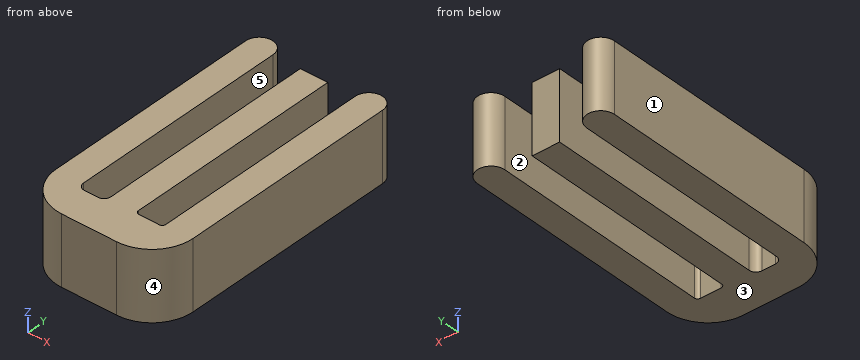
Autodesk Fusion 360 part; units mm, degrees
sketch "Sketch1" plane through (0, 0, 0) normal (0, 0, 1) x (1, 0, 0)
  line L0 (0, 0) -> (200, 0)
  line L1 (200, 0) -> (200, 200)
  line L2 (200, 200) -> (0, 200)
  line L3 (0, 200) -> (0, 0)
  line L4 (52.8009, 30) -> (52.8009, 190)
  line L5 (72.8009, 190) -> (72.8009, 30)
  line L6 (112.8009, 190) -> (112.8009, 30)
  line L7 (132.8009, 190) -> (132.8009, 30)
  line L8 (152.8009, 190) -> (152.8009, 30)
  line L9 (52.8009, 190) -> (152.8009, 190) construction
  arc A0 (72.8009, 190) -> (52.8009, 190) centre (62.8009, 190) ccw
  arc A1 (152.8009, 190) -> (132.8009, 190) centre (142.8009, 190) ccw
  line L10 (92.8009, 190) -> (92.8009, 30)
  arc A2 (72.8009, 30) -> (92.8009, 30) centre (82.8009, 30) ccw construction
  arc A3 (112.8009, 30) -> (132.8009, 30) centre (122.8009, 30) ccw construction
  arc A4 (112.8009, 190) -> (92.8009, 190) centre (102.8009, 190) ccw construction
  arc A5 (52.8009, 30) -> (82.8009, 0) centre (82.8009, 30) ccw
  line L11 (92.8009, 190) -> (112.8009, 190)
  arc A6 (72.8009, 30) -> (77.8009, 25) centre (77.8009, 30) ccw
  arc A7 (87.8009, 25) -> (92.8009, 30) centre (87.8009, 30) ccw
  arc A8 (112.8009, 30) -> (115.3009, 27.5) centre (115.3009, 30) ccw
  arc A9 (130.3009, 27.5) -> (132.8009, 30) centre (130.3009, 30) ccw
  line L12 (77.8009, 25) -> (87.8009, 25)
  line L13 (115.3009, 27.5) -> (130.3009, 27.5)
  line L14 (82.8009, 0) -> (122.8009, 0)
  line L15 (52.8009, 30) -> (152.8009, 30) construction
  arc A10 (122.8009, 0) -> (152.8009, 30) centre (122.8009, 30) ccw
  dimension "d1" = 200
  dimension "d2" = 200
  dimension "d3" = 20
  dimension "d4" = 5
  dimension "d5" = 2.5
  dimension "d6" = 62.8009
extrude "Extrude2" add sketch "Sketch1" along normal blind 50 contours L0 L4 L5 L6 L7 L8 A0 A1 L10 A5 L11 A6 A7 A8 A9 L12 L13 L14 A10
The listing builds one solid part. Answer for the finished solid, in the listing's coordinates (mm). Face numbers are marked on the shaded views. A direction names the side the tool comes from. Round coordinates to 2 decimals unless told otherwise and drop trailing zeros. Loops run counter-clockwise (first coordinate to the right, second up) from the corner with the lowest first, then second, coordinate; pieces in that order, holes last.
Q1. Which of the six approach directions +Z, -Z, +X, -X, +Y, -Y give full straight-line access (tool end or side, diameter ignored) to the marked faces 4 and 5?
Q2. Section A-A, the plane y = 59 is taken. Determine the outline of the cut face in (x, z).
Q3. Find the intervals of material crossed by line 1 (X direction, y = 36, z = 48.5); line 2 (Y direction, x = 105.5, z = 18.5); line 3 (Y direction, x = 121.5, z = 3), in increasing order.
Q4. Given pin 1 Ø2 at (x, z) = (127, 39) entering from +Y; pin 2 Ø6 at (x, z) = (87.5, 15.5) entering from +Y; pin 3 Ø5 at (x, z) = (83, 36.5) entering from +Y, each flat-ended and moving along its own axis, determine where each tip first touches the part or whether it passes through.
Q5. Section D-D, the plane x = 143.5 is taken. Determine the outline of the cut face in (y, z).
Q6. For a pull along X with two mould halves and no side action, classify the marked faces 1, 2 and 3 as released by +X, released by -X, zero draft, split by the parting line, or undercut.
Q7. Section B-B, the plane z = 20 is taken. Determine the outline of the cut face in (x, y), then the cut area to 3 significant figures.
Q8. Section C-C, the plane x = 106 is taken. Determine the outline of the cut face in (y, z).
Completed:
1. face 4: +Z, -Z, +X, -Y
1. face 5: +Z, -Z, +Y
2. outline: (52.8, 0) - (72.8, 0) - (72.8, 50) - (52.8, 50) - close; (92.8, 0) - (112.8, 0) - (112.8, 50) - (92.8, 50) - close; (132.8, 0) - (152.8, 0) - (152.8, 50) - (132.8, 50) - close
3. line 1: x = 52.8 to 72.8, 92.8 to 112.8, 132.8 to 152.8
3. line 2: y = 0 to 190
3. line 3: y = 0 to 27.5
4. pin 1: stops at y = 27.5
4. pin 2: stops at y = 25.79
4. pin 3: stops at y = 25
5. outline: (8.28, 0) - (199.98, 0) - (199.98, 50) - (8.28, 50) - close
6. face 1: released by -X
6. face 2: undercut
6. face 3: zero draft
7. outline: (52.8, 30) arc R30 ccw to (82.8, 0) - (122.8, 0) arc R30 ccw to (152.8, 30) - (152.8, 190) arc R10 ccw to (132.8, 190) - (132.8, 30) arc R2.5 cw to (130.3, 27.5) - (115.3, 27.5) arc R2.5 cw to (112.8, 30) - (112.8, 190) - (92.8, 190) - (92.8, 30) arc R5 cw to (87.8, 25) - (77.8, 25) arc R5 cw to (72.8, 30) - (72.8, 190) arc R10 ccw to (52.8, 190) - close
7. area: 12,400 mm2
8. outline: (0, 0) - (190, 0) - (190, 50) - (0, 50) - close
